Can you work these out from the model? Positions are in its coordinate system, mm. Face numbers are marked on the shaded views. A direction names the side the tool comes from. Coordinates: 2 decimals unless noted, no trailing zeros. Order: outer loops, then holes, each group sorted by start corner. A loop starts at its lowest first (then second) coordinate and runs counter-clockwise, first axis right, second up. Notation, with made-up numbers: (-35, 21) -> (17, 21) arc R11 cw to (17, 29) -> close; hole circle Ø5 at (59.25, 50). An arc over 180 degrees is marked (long way). Return JSON: item names as keys, results as strings. Group by question number.
1) For pin 1 (5 mm diameter, centred on x = -11, y = 15.5, fed in from -Z); pin 2 (2.5 mm diameter, centred on x = -11, y = 15.5, fed in from -Z); pin 3 (1 mm diameter, centred on x = 7, z = -14.5, fed in from +Y); pin 4 (1 mm diameter, centred on x = 7.5, z = 1.5, fed in from +Y), each with a flat end and sliding along its axis, tell me the tip position at first contact or that it passes through.
2) For the marked faces 5 and 6, which set-ups out of +Z, -Z, +X, -X, +Y, -Y let a thin tool reach every point of the face, with its end or its side?
3) If we section it at B-B, the plane y = 8.75: Please give me the cut outline in (x, z), then the cut area to 3 significant figures.
4) If we section it at D-D, the plane x = 6.5: Please give me the cut outline in (y, z).
5) Thinking about a two-plate mould opening in X: for the marked faces 1, 2, 3 and 4, which applies, +X half, -X half, draft (parallel to the pull), parting line (faces both ways), or undercut?
6) If we section it at C-C, the plane z = 18: Please give me the cut outline in (x, y) (3 decimals), then the cut area to 3 significant figures.
7) If I drill on probe 1 along X at (y, z) = (15.5, 18) (3 decimals); probe 2 along Z at (x, y) = (3.5, 18.5); probe 3 along Z at (x, y) = (12.5, 5.5), over which ranges is the centre line in solid material (lowest first)? Write a range as from..to.
8) If we section it at A-A, the plane y = 23.75: Please give me the cut outline in (x, z), then the cut area to 3 significant figures.
from build123d import *

# Parameters (mm, degrees)
SKETCH1_W               = 36
SKETCH1_H               = 30
BASE_PLATE_DEPTH        = 7.5
SKETCH2_W               = 36
SKETCH2_H               = 6
SIDE_WALLS_DEPTH        = 25.5
SKETCH4_R               = 1.25
M2_SCREWS_DEPTH         = 25.5
SKETCH6_W               = 5
SKETCH6_H               = 30
RETURN_STOPPER_DEPTH    = 4.5
SKETCH9_W               = 10
SKETCH9_H               = 15
BOSS_EXTRUDE1_DEPTH     = 4.5
SKETCH7_R               = 6.25
MAGNET_POCKET_DEPTH     = 11
SKETCH8_R               = 2
M2_SCREW_HEAD_DEPTH     = 1.5
M3_ACHSE_DEPTH          = 48.647140523
M3_ACHSE_DEPTH_BACK     = 48.647140523
SKETCH5_R               = 1.625
FILLET1_R               = 1.5
LEAVER_SPACE_DEPTH      = 30.25
LEAVER_SPACE_DEPTH_BACK = 0.25
SKETCH11_W              = 23
SKETCH11_H              = 13.5
SKETCH12_W              = 18
SKETCH12_H              = 4.5
MORE_SPACE_LEFT_DEPTH   = 0.25
SKETCH13_W              = 18
SKETCH13_H              = 4.5
MORE_SPACE_RIGHT_DEPTH  = 0.25
FILLET2_R               = 0.75
FILLET3_R               = 0.75
FILLET4_R               = 0.75
FILLET5_R               = 0.5


with BuildPart() as part:
    # Sketch1 → Base Plate (new body)
    with BuildSketch(Plane(origin=(0, 0, 0), x_dir=(1, 0, 0), z_dir=(0, 1, 0))):
        Rectangle(SKETCH1_W, SKETCH1_H)
    extrude(amount=BASE_PLATE_DEPTH)

    # Sketch2 → Side Walls (add)
    with BuildSketch(Plane.XZ):
        with Locations((0, -18)):
            Rectangle(SKETCH2_W, SKETCH2_H)
        with Locations((0, 18)):
            Rectangle(SKETCH2_W, SKETCH2_H)
    extrude(amount=-SIDE_WALLS_DEPTH)

    # Sketch4 → M2 Screws (cut)
    with BuildSketch(Plane(origin=(0, 25.5, 0), x_dir=(1, 0, 0), z_dir=(0, 1, 0))):
        with Locations(Location((-13, -18, 0), (0, 0, 270))):
            Circle(SKETCH4_R)
        with Locations(Location((13, -18, 0), (0, 0, 270))):
            Circle(SKETCH4_R)
        with Locations(Location((13, 18, 0), (0, 0, 270))):
            Circle(SKETCH4_R)
        with Locations(Location((-13, 18, 0), (0, 0, 270))):
            Circle(SKETCH4_R)
    extrude(amount=-M2_SCREWS_DEPTH, mode=Mode.SUBTRACT)

    # Sketch6 → Return Stopper (add)
    with BuildSketch(Plane(origin=(0, 7.5, 0), x_dir=(1, 0, 0), z_dir=(0, 1, 0))):
        with Locations((15.5, 0)):
            Rectangle(SKETCH6_W, SKETCH6_H)
    extrude(amount=RETURN_STOPPER_DEPTH)

    # Sketch9 → Boss-Extrude1 (add)
    with BuildSketch(Plane(origin=(0, 7.5, 0), x_dir=(1, 0, 0), z_dir=(0, 1, 0))):
        with Locations((8, 0)):
            Rectangle(SKETCH9_W, SKETCH9_H)
    extrude(amount=BOSS_EXTRUDE1_DEPTH)

    # Sketch7 → Magnet Pocket (cut)
    with BuildSketch(Plane(origin=(0, 0, 0), x_dir=(-1, 0, 0), z_dir=(0, 1, 0))):
        with Locations(Location((-11, 0, 0), (0, 0, 270))):
            Circle(SKETCH7_R)
    extrude(amount=MAGNET_POCKET_DEPTH, mode=Mode.SUBTRACT)

    # Sketch8 → M2 Screw Head (cut)
    with BuildSketch(Plane.XZ):
        with Locations(Location((13, -18, 0), (0, 0, 270))):
            Circle(SKETCH8_R)
        with Locations(Location((-13, -18, 0), (0, 0, 270))):
            Circle(SKETCH8_R)
        with Locations(Location((13, 18, 0), (0, 0, 270))):
            Circle(SKETCH8_R)
        with Locations(Location((-13, 18, 0), (0, 0, 270))):
            Circle(SKETCH8_R)
    extrude(amount=-M2_SCREW_HEAD_DEPTH, mode=Mode.SUBTRACT)

    # Sketch5 → M3 Achse (cut, two sides: drawn at the far end of the back side and taken through both)
    with BuildSketch(Plane.XY.offset(-15).offset(-M3_ACHSE_DEPTH_BACK)):
        with Locations((-11, 15.5)):
            Circle(SKETCH5_R)
    extrude(amount=M3_ACHSE_DEPTH + M3_ACHSE_DEPTH_BACK, mode=Mode.SUBTRACT)

    # Fillet1
    fillet1_edges = [part.edges().sort_by_distance(p)[0] for p in [
        (3, 12, 0),
    ]]
    fillet(fillet1_edges, radius=FILLET1_R)

    # Sketch11 → Leaver Space (cut, two sides: drawn at the far end of the back side and taken through both)
    with BuildSketch(Plane.XY.offset(-15).offset(-LEAVER_SPACE_DEPTH_BACK)):
        with Locations((6.5, 18.75)):
            Rectangle(SKETCH11_W, SKETCH11_H)
    extrude(amount=LEAVER_SPACE_DEPTH + LEAVER_SPACE_DEPTH_BACK, mode=Mode.SUBTRACT)

    # Sketch12 → More Space left (cut)
    with BuildSketch(Plane.XY.offset(-15)):
        with Locations((4, 9.75)):
            Rectangle(SKETCH12_W, SKETCH12_H)
    extrude(amount=-MORE_SPACE_LEFT_DEPTH, mode=Mode.SUBTRACT)

    # Sketch13 → More Space right (cut)
    with BuildSketch(Plane(origin=(0, 0, 15), x_dir=(-1, 0, 0), z_dir=(0, 0, -1))):
        with Locations((-4, 9.75)):
            Rectangle(SKETCH13_W, SKETCH13_H)
    extrude(amount=-MORE_SPACE_RIGHT_DEPTH, mode=Mode.SUBTRACT)

    # Fillet2
    fillet2_edges = [part.edges().sort_by_distance(p)[0] for p in [
        (0, 0, -21),
    ]]
    fillet(fillet2_edges, radius=FILLET2_R)

    # Fillet3
    fillet3_edges = [part.edges().sort_by_distance(p)[0] for p in [
        (0, 0, 21),
    ]]
    fillet(fillet3_edges, radius=FILLET3_R)

    # Fillet4
    fillet4_edges = [part.edges().sort_by_distance(p)[0] for p in [
        (-18, 13.125, 21),
        (-18, 0, 0),
        (-18, 0.219669914, -20.780330086),
        (-18, 0.219669914, 20.780330086),
        (-18, 13.125, -21),
    ]]
    fillet(fillet4_edges, radius=FILLET4_R)

    # Fillet5
    fillet5_edges = [part.edges().sort_by_distance(p)[0] for p in [
        (18, 13.125, 21),
        (18, 0.219669914, -20.780330086),
        (18, 0, 0),
        (18, 0.219669914, 20.780330086),
        (18, 13.125, -21),
    ]]
    fillet(fillet5_edges, radius=FILLET5_R)


solid = part.part
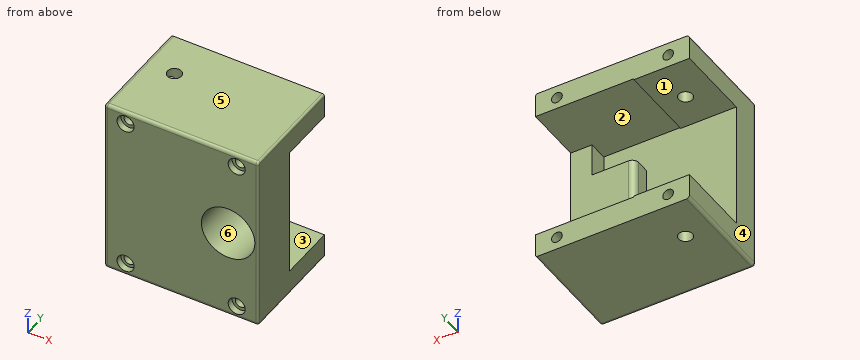
Result sheet:
{
 "1": {"pin 1": "stops at z = -21", "pin 2": "passes through", "pin 3": "stops at y = 7.5", "pin 4": "stops at y = 12"},
 "2": {"face 5": "+Z, +X, -X, +Y, -Y", "face 6": "-Y"},
 "3": {"outline": "(-18, -20.25) arc R0.75 ccw to (-17.25, -21) -> (17.5, -21) arc R0.5 ccw to (18, -20.5) -> (18, 20.5) arc R0.5 ccw to (17.5, 21) -> (-17.25, 21) arc R0.75 ccw to (-18, 20.25) -> (-18, 15) -> (-5, 15) -> (-5, 15.25) -> (13, 15.25) -> (13, 7.5) -> (3, 7.5) -> (3, -7.5) -> (13, -7.5) -> (13, -15.25) -> (-5, -15.25) -> (-5, -15) -> (-18, -15) -> close; hole circle Ø2.5 at (-13, -18); hole circle Ø2.5 at (-13, 18); hole circle Ø12.5 at (11, 0); hole circle Ø2.5 at (13, -18); hole circle Ø2.5 at (13, 18)", "area": "580 mm2"},
 "4": {"outline": "(0, -20.25) arc R0.75 ccw to (0.75, -21) -> (25.5, -21) -> (25.5, -15.25) -> (7.5, -15.25) -> (7.5, -7.5) -> (12, -7.5) -> (12, 7.5) -> (7.5, 7.5) -> (7.5, 15.25) -> (25.5, 15.25) -> (25.5, 21) -> (0.75, 21) arc R0.75 ccw to (0, 20.25) -> (0, 4.34) -> (11, 4.34) -> (11, -4.34) -> (0, -4.34) -> close"},
 "5": {"face 1": "draft", "face 2": "undercut", "face 3": "undercut", "face 4": "-X half"},
 "6": {"outline": "(-18, 0.75) arc R0.75 ccw to (-17.25, 0) -> (-15, 0) -> (-15, 1.5) -> (-14.25, 1.5) -> (-14.25, 25.5) -> (-18, 25.5) -> close; (-11.75, 1.5) -> (-11, 1.5) -> (-11, 0) -> (11, 0) -> (11, 1.5) -> (11.75, 1.5) -> (11.75, 25.5) -> (-11.75, 25.5) -> (-11.75, 16.942) arc R1.625 cw (long way) to (-11.75, 14.058) -> close; (14.25, 1.5) -> (15, 1.5) -> (15, 0) -> (17.5, 0) arc R0.5 ccw to (18, 0.5) -> (18, 25.5) -> (14.25, 25.5) -> close", "area": "779 mm2"},
 "7": {"probe 1": "x = -18..-14.25, -9.375..11.75, 14.25..18", "probe 2": "z = -21..-15.25, 15.25..21", "probe 3": "z = -21..-19.15, -16.85..-6.07, 6.07..16.85, 19.15..21"},
 "8": {"outline": "(-18, -20.25) arc R0.75 ccw to (-17.25, -21) -> (17.5, -21) arc R0.5 ccw to (18, -20.5) -> (18, -15.25) -> (-5, -15.25) -> (-5, -15) -> (-18, -15) -> close; (-18, 15) -> (-5, 15) -> (-5, 15.25) -> (18, 15.25) -> (18, 20.5) arc R0.5 ccw to (17.5, 21) -> (-17.25, 21) arc R0.75 ccw to (-18, 20.25) -> close; hole circle Ø2.5 at (-13, -18); hole circle Ø2.5 at (-13, 18); hole circle Ø2.5 at (13, -18); hole circle Ø2.5 at (13, 18)", "area": "401 mm2"}
}
